Check sheet for the modelled part. Datum: model origin and axes. Units: mm. A direction names the side the tool comes from. Give positions to 0.01 mm unless a question says otherwise; leave off trailing zeros. Write each loop counter-clockwise with the first axis right and the second up, starting at its lowest first coordinate (ties: lowest second). Pieces come first, ordered by that corner, then holes. Notation, with made-up numbers: (60, -16.75) -> (99, -16.75) arc R32 ccw to (99, 19.25) -> close; hole circle Ø3 at (70, -15.75). An arc over 180 degrees is marked (long way). Return JSON: item names as keys, results as strings.
from build123d import *

# Parameters (mm, degrees)
F1_DEPTH = 1.5


with BuildPart() as f1:
    # F0 (on Front) → F1 (new body, symmetric)
    with BuildSketch(Plane.XZ):
        Polygon((7, 0), (0, 0), (0, -7), (3, -7), (3, -17), (0, -17), (0, -24), (3, -24), (3, -34), (0, -34), (0, -41), (7, -41), (7, -44), (17, -44), (17, -41), (19.25, -41), (19.25, -34.5), (18.5, -34.5), (18.5, -32.5), (19.25, -32.5), (19.25, -29), (21.75, -29), (21.75, -32.5), (22.5, -32.5), (22.5, -34.5), (21.75, -34.5), (21.75, -41), (24, -41), (24, -44.073563), (34, -44.073563), (34, -41), (41, -41), (41, -34), (38, -34), (38, -24), (41, -24), (41, -17), (38, -17), (38, -7), (41, -7), (41, 0), (34, 0), (34, 3.073563), (24, 3.073563), (24, 0), (21.75, 0), (21.75, -6.5), (22.5, -6.5), (22.5, -8.5), (21.75, -8.5), (21.75, -12), (19.25, -12), (19.25, -8.5), (18.5, -8.5), (18.5, -6.5), (19.25, -6.5), (19.25, 0), (17, 0), (17, 3), (7, 3), align=None)
    extrude(amount=F1_DEPTH, both=True)


solid = f1.part
(1) Thickness scan on L1, parallel to Z at x = 22, y = -0.55; L2, parallel to X at y = 1.45, z = -3.5; L3, parallel to Z at x = 15, y = 0.55. Record the ranges inside material, lowest first.
Reply:
{"L1": "-41 to -34.5, -32.5 to -8.5, -6.5 to 0", "L2": "0 to 19.25, 21.75 to 41", "L3": "-44 to 3"}
(2) Set-up check for faces 4 (the flat face through (38, 0, 0)), 5 (the flat face through (21.75, 0, -10)), 6 (the flat face through (22.5, 0, -7)): record each of +Z, -Z, +X, -X, +Y, -Y from which the full face is reachable in a straight line by a thin tool's end or side.
Reply:
{"face 4": "+Z, +X, +Y, -Y", "face 5": "+Z, +Y, -Y", "face 6": "+Y, -Y"}
(3) Depth check by flat-ended pin: pin 1 Ø1.5 at (x, y) = (1.5, -0.5) entering from -Z; pin 2 Ø1.5 at (y, z) = (-0.5, -10) entering from +X. Enter the tip coordinate at first touch or a pass-through.
Reply:
{"pin 1": "z = -41", "pin 2": "x = 38"}
(4) Release check for a two-part mould opening along X. For faces 1 (the flat face through (4, 0, 0)), 2 (the flat face through (18, 0, -41)), 3 (the flat face through (41, 0, -4)) record: pulls with the +X half, pulls with the -X half, needs draft (parallel to the pull), parting line crosses it, or undercut.
Reply:
{"face 1": "needs draft", "face 2": "undercut", "face 3": "pulls with the +X half"}
(5) Cross-section at C-C on x = 5.5. Enter the section's corners in (y, z).
Reply:
{"outline": "(-1.5, -41) -> (1.5, -41) -> (1.5, 0) -> (-1.5, 0) -> close"}
(6) Cross-section at A-A on z = -37. Enter the section's corners in (x, y).
Reply:
{"outline": "(0, -1.5) -> (19.25, -1.5) -> (19.25, 1.5) -> (0, 1.5) -> close; (21.75, -1.5) -> (41, -1.5) -> (41, 1.5) -> (21.75, 1.5) -> close"}
(7) Cross-section at B-B on z = -27. Enter the section's corners in (x, y).
Reply:
{"outline": "(3, -1.5) -> (38, -1.5) -> (38, 1.5) -> (3, 1.5) -> close"}
